Solid Edge part; units mm, degrees
sketch "Sketch1" plane through (0, 0, 0) normal (0, 0, 1) x (1, 0, 0)
  line L0 (0, 0) -> (0, 12.7)
  line L1 (0, 12.7) -> (107.95, 12.7)
  line L2 (107.95, 25.4) -> (107.95, 12.7)
  line L3 (107.95, 25.4) -> (184.15, 25.4)
  line L4 (184.15, 25.4) -> (184.15, 12.7)
  line L5 (184.15, 12.7) -> (292.1, 12.7)
  line L6 (292.1, 12.7) -> (292.1, 0)
  line L7 (292.1, 0) -> (0, 0)
  dimension "D1" = 292.1
  dimension "D2" = 107.95
  dimension "D3" = 107.95
  dimension "D4" = 184.15
extrude "Protrusion1" add sketch "Sketch1" along normal blind 1.524
sketch "Sketch2" plane through (146.05, 12.7, 1.524) normal (0, 0, 1) x (1, 0, 0)
  line L0 (-146.05, 0) -> (-146.05, -203.2)
  line L1 (-146.05, -203.2) -> (-139.7, -203.2)
  line L2 (-139.7, -203.2) -> (-139.7, 0)
  line L3 (-139.7, 0) -> (-146.05, 0)
  dimension "D1" = 146.05
  dimension "D2" = 146.05
extrude "Protrusion_2" add sketch "Sketch2" against normal blind 1.524
pattern_linear "Pattern1" count 4 spacing 95.25 along (1, 0, 0) of "Protrusion_2"
fillet "Round_1" radius 9.525 10 edges at (0, 12.7, 0.762) (6.35, 0, 0.762) (95.25, 0, 0.762) (101.6, 0, 0.762) (107.95, 12.7, 0.762) (184.15, 12.7, 0.762) (190.5, 0, 0.762) (196.85, 0, 0.762) (285.75, 0, 0.762) (292.1, 12.7, 0.762)
fillet "Round_2" radius 3.175 8 edges at (0, -190.5, 0.762) (6.35, -190.5, 0.762) (95.25, -190.5, 0.762) (101.6, -190.5, 0.762) (190.5, -190.5, 0.762) (196.85, -190.5, 0.762) (285.75, -190.5, 0.762) (292.1, -190.5, 0.762)
hole "Hole_1" at (171.45, 12.7, 1.524) direction (0, 0, -1) diameter 4.826 end up to next
hole "Hole1" at (120.65, 12.7, 1.524) direction (0, 0, -1) diameter 4.826 end up to next
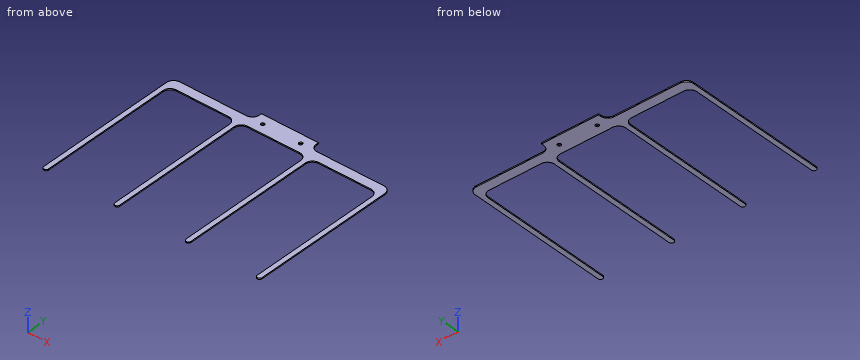
CAD build for the part. Positions are in the model's coordinates, mm. Coordinates: 2 decimals unless noted, no trailing zeros. Order: outer loops, then holes, each group sorted by start corner. A loop starts at its lowest first (then second) coordinate and runs counter-clockwise, first axis right, second up. Notation, with made-up numbers: M 83.5,-10.75 L 119.5,-10.75 A23 cw 119.5,17.25 Z; hole C 73,57 d7. An arc over 180 degrees is marked long. Answer as CSV lines item,"result".
1) Cut at B-B (z = 1). Give the number of separate pieces and of enclosed holes in the cut face, then the cut area to 3 significant figures.
Verdict:
separate pieces,"1"
enclosed holes,"2"
area,"9,580 mm2"
2) Drill centre lines: L1, parallel to X at y = -157.5, z = 1.2; L2, parallel to Y at x = 171.45, z = 0.4; L3, parallel to X at y = 10.5, z = 1.2. Where is each one in solid material? Low to high. Write a range as from..to.
Verdict:
L1,"0..6.35, 95.25..101.6, 190.5..196.85, 285.75..292.1"
L2,"0..10.29, 15.11..25.4"
L3,"3.44..119.66, 121.64..170.46, 172.44..288.66"
3) Cut at D-D (x = 212.5). List the corners of the cut face in (y, z).
Verdict:
outline,"M 0,0 L 12.7,0 L 12.7,1.52 L 0,1.52 Z"
4) Cut at C-C (y = -6). List the corners of the cut face in (x, z), then the cut area to 3 significant figures.
Verdict:
outline,"M 0,0 L 7.03,0 L 7.03,1.52 L 0,1.52 Z; M 94.57,0 L 102.28,0 L 102.28,1.52 L 94.57,1.52 Z; M 189.82,0 L 197.53,0 L 197.53,1.52 L 189.82,1.52 Z; M 285.07,0 L 292.1,0 L 292.1,1.52 L 285.07,1.52 Z"
area,"44.9 mm2"
5) Flat gauge pins, fed straight in: P1, Ø4.5, axis at x = 171.45, y = 12.7, coming from the +Z side; P2, Ø0.5, axis at y = 23.5, z = 0.5, coming from the -X side; P3, Ø0.5, axis at y = 23.5, z = 1, coming from the +X side. Where does each tip first touch, or does it go through?
Verdict:
P1,"through"
P2,"x = 107.95"
P3,"x = 184.15"
6) Cut at A-A (y = -36.5). List the corners of the cut face in (x, z).
Verdict:
outline,"M 0,0 L 6.35,0 L 6.35,1.52 L 0,1.52 Z; M 95.25,0 L 101.6,0 L 101.6,1.52 L 95.25,1.52 Z; M 190.5,0 L 196.85,0 L 196.85,1.52 L 190.5,1.52 Z; M 285.75,0 L 292.1,0 L 292.1,1.52 L 285.75,1.52 Z"
